Design review of the part built by this model. Coordinates are the model's own, in mm. Face numbers are marked on the shaded views. A direction names the side the tool comes from. Coordinates: 2 decimals unless noted, no trailing zeros. Write each loop counter-clockwise with the first axis right and the second up, starting at its lowest first coordinate (ties: lowest second). Pieces come first, ordered by that corner, then holes.
Q1. The part is to be moulded in two halves that separate along Y. For the marked faces 1, 2 and 3, say which applies: +Y half, -Y half, draft (parallel to the pull), parting line (faces both ways), or undercut.
Q2. Add section D-D, the plane y = -21. Give the boundary of the cut face in (x, z), plus the area to 3 significant figures.
Q3. To check wall thickness, follow probe 1 along Y at (x, z) = (0, 31.25); probe 2 along Y at (x, z) = (0, 49.75); probe 3 along Z at (x, y) = (19, 7). State the ranges of each line that lie inside material, in increasing order.
Q4. Clearance check with flat-ended pins moving along their axes: pin 1 Ø1.5 at (x, z) = (-24.5, 18.5) entering from +Y; pin 2 Ø4 at (y, z) = (20, 30) entering from +X; pin 3 Ø5 at (x, z) = (-21, 20.5) entering from -Y; pin 4 Ø1.5 at (x, y) = (22.5, -21) entering from -Z. State where each tip first meets the part, or that it passes through.
Q5. Add section C-C, the plane z = 24.5. Give the boundary of the cut face in (x, y), plus the area to 3 significant figures.
Q6. Machinability: for the marked faces 4 and 5, which of the approach directions +Z, -Z, +X, -X, +Y, -Y give a long, thin tool a straight path to every point of the face, cutting with its end or side? Answer none if there is none.
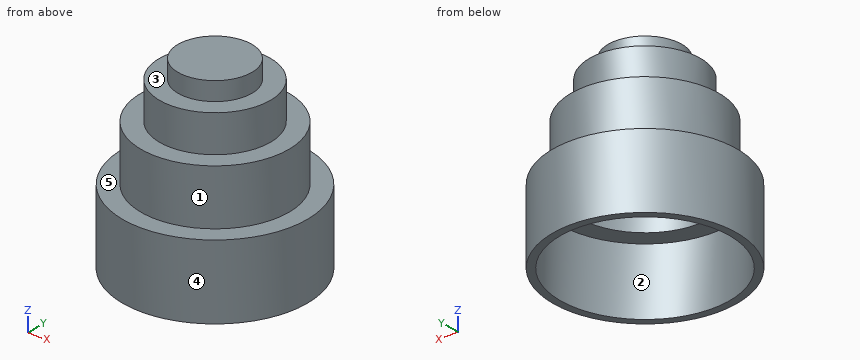
from build123d import *

# Parameters (mm, degrees)
F0_R     = 31.75
F1_DEPTH = 25.4
F2_R     = 25.4
F3_DEPTH = 19.05
F4_R     = 19.05
F5_DEPTH = 12.7
F6_R     = 12.7
F7_DEPTH = 6.35
F8_T     = -2.54


with BuildPart() as f1:
    # F0 (on Top) → F1 (new body)
    with BuildSketch(Plane.XY):
        Circle(F0_R)
    extrude(amount=F1_DEPTH)

    # F2 (on face) → F3 (join)
    with BuildSketch(Plane.XY.offset(25.4)):
        Circle(F2_R)
    extrude(amount=F3_DEPTH)

    # F4 (on face) → F5 (join)
    with BuildSketch(Plane.XY.offset(44.45)):
        Circle(F4_R)
    extrude(amount=F5_DEPTH)

    # F6 (on face) → F7 (join)
    with BuildSketch(Plane.XY.offset(57.15)):
        Circle(F6_R)
    extrude(amount=F7_DEPTH)

    # F8
    f8_openings = [f1.faces().sort_by_distance(p)[0] for p in [
        (0, 0, 0),
    ]]
    offset(amount=F8_T, openings=f8_openings, kind=Kind.INTERSECTION)


solid = f1.part
Here are the results:
1. face 1: parting line
1. face 2: undercut
1. face 3: draft
2. outline: (-23.81, 0) - (-20.3, 0) - (-20.3, 22.86) - (-9.03, 22.86) - (-9.03, 41.91) - (9.03, 41.91) - (9.03, 22.86) - (20.3, 22.86) - (20.3, 0) - (23.81, 0) - (23.81, 25.4) - (14.29, 25.4) - (14.29, 44.45) - (-14.29, 44.45) - (-14.29, 25.4) - (-23.81, 25.4) - close
2. area: 482 mm2
3. probe 1: y = -25.4 to -22.86, 22.86 to 25.4
3. probe 2: y = -19.05 to -16.51, 16.51 to 19.05
3. probe 3: z = 41.91 to 44.45
4. pin 1: stops at y = 21.07
4. pin 2: stops at x = 17.92
4. pin 3: stops at y = -25.8
4. pin 4: stops at z = 0
5. outline: circle Ø63.5 at (0, 0); hole circle Ø45.72 at (0, 0)
5. area: 1,530 mm2
6. face 4: +Z, -Z
6. face 5: +Z
